CAD build for the part. Positions are in the model's coordinates, mm. Face numbers are marked on the shaded views. A direction names the side the tool comes from. Coordinates: 2 decimals unless noted, no trailing zeros. Loops run counter-clockwise (first coordinate to the right, second up) from the corner with the lowest first, then second, coordinate; pieces in that order, holes last. Notation, with made-up numbers: (69.5, -32) -> (108.5, -32) arc R14 cw to (108.5, -14) -> close; hole circle Ø9 at (15.25, -33). An arc over 180 degrees is marked (long way). Write item = value, one per line. Start each with the question number.
(1) Flat gauge pins, fed straight in: P1, Ø1, axis at y = 0.5, z = 18, coming from the -X side; P2, Ø2, axis at x = 3, y = 3.5, coming from the +Z side; P3, Ø2, axis at x = -3, z = 13.5, coming from the +Y side. Where does each tip first touch, or does it go through?
(2) Drill centre lines: line 1 (Y direction, x = 0, z = 6.75); line 2 (Z direction, x = 1.75, y = 2.5); line 3 (Y direction, x = -0.5, z = 10.25). Where is each one in solid material? Low to high. Write a range as from..to.
(3) Tool access for the marked faces 1, 2, 3, 4 and 5: list every direction of +Z, -Z, +X, -X, +Y, -Y with a clear straight run to the whole face (end or side of a thin tool).
(4) Pull direction Z, two halves, no side cores. Call the marked faces 6, 7, 8 and 9: +Z half, -Z half, draft (parallel to the pull), parting line (faces both ways), or undercut.
(5) Band-saw the part on B-B (z = 7.25). Write the cut outline in (x, y).
(6) Band-saw the part on A-A (z = 10.25). Write the cut outline in (x, y), and give its area (3 significant figures).
(7) Band-saw the part on C-C (z = 20.75). Write the cut outline in (x, y), and give its area (3 significant figures).
Autodesk Inventor part; units mm, degrees
ref_plane "YZ Plane" through (0, 0, 0) normal (1, 0, 0) x (0, 1, 0)
ref_plane "XZ Plane" through (0, 0, 0) normal (0, 1, 0) x (-1, 0, 0)
ref_plane "XY Plane" through (0, 0, 0) normal (0, 0, 1) x (1, 0, 0)
sketch "Sketch1" plane through (0, 0, 0) normal (0, 0, 1) x (1, 0, 0)
  circle A0 centre (0, 0) radius 2.5
  circle A1 centre (0, 0) radius 5
  dimension "d0" = 5
  dimension "d1" = 10
extrude "Extrusion1" add sketch "Sketch1" along normal blind 10
sketch "Sketch2" plane through (0, 0, 10) normal (0, 0, 1) x (1, 0, 0)
  circle A0 centre (0, 0) radius 5
  circle A1 centre (0, 0) radius 5
  line L0 (-4.899, 1) -> (4.899, 1)
  line L1 (-4.899, -1) -> (4.899, -1)
  line L2 (-1, 4.899) -> (-1, -4.899)
  line L3 (1, -4.899) -> (1, 4.899)
  point P0 (1, 1)
  point P1 (-1, 1)
  point P2 (-1, -1)
  point P3 (1, -1)
  dimension "d4" = 1
  dimension "d5" = 1
  dimension "d6" = 1
  dimension "d7" = 1
extrude "Extrusion2" add sketch "Sketch2" along normal blind 2 contours A0 L1 L3 L0 | L3 L0 L2 A0 | L3 L1 L2 L0 | A0 L2 L1 L3 | L2 L1 A0 L0
sketch "Sketch3" plane through (0, 0, 12) normal (0, 0, 1) x (1, 0, 0)
  circle A0 centre (0, 0) radius 5
  dimension "d11" = 10
extrude "Extrusion3" add sketch "Sketch3" along normal blind 2
chamfer "Chamfer1" distance 1 angle 45 1 edges at (-5, 0, 0)
sketch "Sketch4" plane through (0, 0, 10) normal (0, 0, -1) x (-1, 0, 0)
  circle A0 centre (0, 0) radius 2
  dimension "d17" = 4
extrude "Extrusion4" cut sketch "Sketch4" against normal blind 2
fillet "Fillet2" radius 0.5 8 edges at (-1, 1.7321, 11) (-1, -1.7321, 11) (-1.7321, -1, 11) (1.7321, -1, 11) (1.7321, 1, 11) (-1.7321, 1, 11) (1, 1.7321, 11) (1, -1.7321, 11)
sketch "Sketch5" plane through (0, 0, 14) normal (0, 0, 1) x (1, 0, 0)
  line L0 (-2.5, 2.5) -> (2.5, 2.5)
  line L1 (2.5, 2.5) -> (2.5, -2.5)
  line L2 (2.5, -2.5) -> (-2.5, -2.5)
  line L3 (-2.5, -2.5) -> (-2.5, 2.5)
  line L4 (-2.5, 2.5) -> (2.5, -2.5) construction
  line L5 (2.5, 2.5) -> (-2.5, -2.5) construction
  point P0 (0, 0)
  dimension "d21" = 5
  dimension "d22" = 5
extrude "Extrusion5" add sketch "Sketch5" along normal blind 8
chamfer "Chamfer2" distance 0.8 angle 45 4 edges at (2.5, 2.5, 18) (-2.5, 2.5, 18) (2.5, -2.5, 18) (-2.5, -2.5, 18)
sketch "Sketch6" plane through (0, 0, 0) normal (1, 0, 0) x (0, 1, 0)
  line L0 (5.5, 13.5) -> (4.5, 13.5)
  line L1 (4.5, 13.5) -> (4.5, 12.5)
  line L2 (4.5, 12.5) -> (5.5, 12.5)
  line L3 (5.5, 12.5) -> (5.5, 13.5)
  line L4 (5, 1) -> (5, 14)
  line L5 (5.5, 13.5) -> (4.5, 12.5) construction
  line L6 (4.5, 13.5) -> (5.5, 12.5) construction
  line L7 (5.5, 6.5) -> (4.5, 6.5)
  line L8 (4.5, 6.5) -> (4.5, 5.5)
  line L9 (4.5, 5.5) -> (5.5, 5.5)
  line L10 (5.5, 5.5) -> (5.5, 6.5)
  line L11 (5.5, 6.5) -> (4.5, 5.5) construction
  line L12 (4.5, 6.5) -> (5.5, 5.5) construction
  line L13 (4.899, 10) -> (4.899, 12)
  line L14 (4.899, 12) -> (1, 12)
  line L15 (4.899, 12) -> (4.899, 14)
  line L16 (4.899, 10) -> (1, 10)
  line L17 (0, -4.4) -> (0, 26.4)
  point P0 (0, 0)
  point P1 (5, 13)
  point P2 (5, 6)
  dimension "d28" = 1
  dimension "d29" = 1
  dimension "d30" = 1
  dimension "d31" = 4
revolve "Revolution1" cut sketch "Sketch6" angle 360 about axis through (0, 0, -10) along (0, 0, 1)
fillet "Fillet3" radius 0.4 4 edges at (0, -4.5, 13.5) (0, -4.5, 6.5) (0, -4.5, 5.5) (0, -4.5, 12.5)
properties part number "VacuumRotor" material "Nylon, molybdenum disulphide"
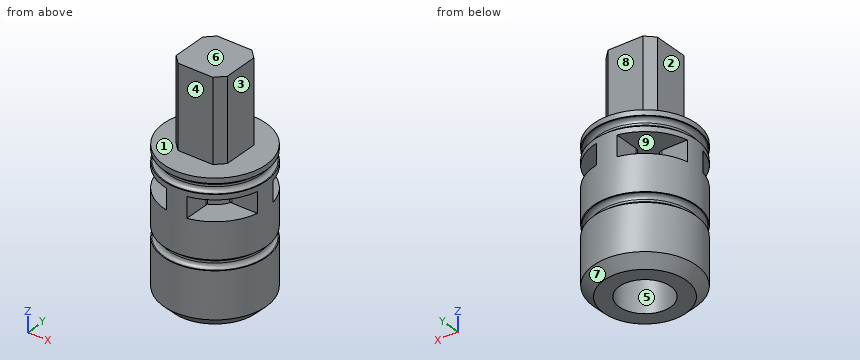
Findings below:
q1.P1 = -2.5
q1.P2 = 14
q1.P3 = 4.58
q2.line_1 = -5..-2.5, 2.5..5
q2.line_2 = 0..10, 12..14
q2.line_3 = -4.97..-1.95, 1.95..4.97
q3.face_1 = +Z
q3.face_2 = +Z, -X, +Y, -Y
q3.face_3 = +Z, +X, +Y, -Y
q3.face_4 = +Z, +X, -X, -Y
q3.face_5 = -Z
q4.face_6 = +Z half
q4.face_7 = -Z half
q4.face_8 = draft
q4.face_9 = undercut
q5.outline = circle Ø10 at (0, 0); hole circle Ø5 at (0, 0)
q6.outline = (-4.9, -1) -> (-2.45, -1) arc R0.5 ccw to (-1.96, -0.4) arc R2 cw to (-1.96, 0.4) arc R0.5 ccw to (-2.45, 1) -> (-4.9, 1) arc R5 ccw to start; (-1, -4.9) arc R5 ccw to (1, -4.9) -> (1, -2.45) arc R0.5 ccw to (0.4, -1.96) arc R2 cw to (-0.4, -1.96) arc R0.5 ccw to (-1, -2.45) -> close; (-1, 2.45) arc R0.5 ccw to (-0.4, 1.96) arc R2 cw to (0.4, 1.96) arc R0.5 ccw to (1, 2.45) -> (1, 4.9) arc R5 ccw to (-1, 4.9) -> close; (1.96, -0.4) arc R0.5 ccw to (2.45, -1) -> (4.9, -1) arc R5 ccw to (4.9, 1) -> (2.45, 1) arc R0.5 ccw to (1.96, 0.4) arc R2 cw to start
q6.area = 23.6 mm²
q7.outline = (-2.5, -1.7) -> (-1.7, -2.5) -> (1.7, -2.5) -> (2.5, -1.7) -> (2.5, 1.7) -> (1.7, 2.5) -> (-1.7, 2.5) -> (-2.5, 1.7) -> close
q7.area = 23.7 mm²
